Autodesk Inventor part; units mm, degrees
ref_plane "YZ Plane" through (0, 0, 0) normal (1, 0, 0) x (0, 1, 0)
ref_plane "XZ Plane" through (0, 0, 0) normal (0, 1, 0) x (-1, 0, 0)
ref_plane "XY Plane" through (0, 0, 0) normal (0, 0, 1) x (1, 0, 0)
sketch "スケッチ1" plane through (0, 0, 0) normal (1, 0, 0) x (0, 1, 0)
  line L0 (0, 0) -> (50.2, 0)
  line L1 (50.2, 0) -> (50.2, -28.2)
  line L2 (50.2, -28.2) -> (0, -28.2)
  line L3 (0, -28.2) -> (0, 0)
  line L4 (50.2, -14.1) -> (0, -14.1)
  line L5 (25.1, -28.2) -> (25.1, 0)
  circle A0 centre (25.1, -14.1) radius 15.3335
  point P0 (19.0745, 0)
  point P1 (19.0745, -28.2)
  point P2 (31.1255, -28.2)
  point P3 (31.1255, 0)
  dimension "d0" = 50.2
  dimension "d1" = 28.2
  dimension "d2" = 30.667
extrude "押し出し1" add sketch "スケッチ1" against normal blind 34
chamfer "面取り1" distance 2.5 angle 45 4 edges at (-17, 50.2, 0) (-17, 50.2, -28.2) (-17, 0, 0) (-17, 0, -28.2)
sketch "スケッチ2" plane through (-34, 0, 0) normal (-1, 0, 0) x (0, 0, 1)
  arc A0 (-28.2, 31.1255) -> (-28.2, 19.0745) centre (-14.1, 25.1) ccw
  circle A1 centre (-14.1, 25.1) radius 19.5
  point P0 (0, 0)
  dimension "d8" = 39
extrude "押し出し2" [suppressed]
sketch "スケッチ3" plane through (-36.375, 22.6, -13.1) normal (-1, 0, 0) x (0, 0, 1)
  arc A0 (-13.1, -14.4444) -> (13.1, -14.4444) centre (0, 0) ccw
  circle A1 centre (0, 0) radius 23
  point P0 (13.1, -22.6)
  dimension "d11" = 46
extrude "押し出し3" [suppressed]
sketch "スケッチ4" plane through (-42.675, 22.6, -13.1) normal (-1, 0, 0) x (0, 0, 1)
  circle A0 centre (0, 0) radius 23
  line L0 (0, 0) -> (19.85, 0)
  line L1 (19.85, 0) -> (19.85, 16.35)
  line L2 (19.85, 16.35) -> (0, 16.35)
  line L3 (0, 16.35) -> (0, 0)
  line L4 (10.6, 22.6) -> (-10.6, 22.6)
  line L5 (19.85, 0) -> (0, 0)
  line L6 (0, 0) -> (0, -14.35)
  line L7 (0, -14.35) -> (19.85, -14.35)
  line L8 (19.85, -14.35) -> (19.85, 0)
  line L9 (-19.85, 0) -> (-19.85, 16.35)
  line L10 (-19.85, 16.35) -> (0, 16.35)
  line L11 (0, -14.35) -> (-19.85, -14.35)
  line L12 (-19.85, -14.35) -> (-19.85, 0)
  point P0 (13.1, -22.6)
  point P1 (17.9744, -14.35)
  point P2 (19.85, -11.618)
  point P3 (19.85, 11.618)
  point P4 (16.1764, 16.35)
  point P5 (-16.1764, 16.35)
  point P6 (-19.85, 11.618)
  point P7 (-19.85, -11.618)
  point P8 (-17.9744, -14.35)
  dimension "d14" = 6.25
  dimension "d16" = 19.85
  dimension "d17" = 30.7
extrude "押し出し4" [suppressed]
sketch "スケッチ5" plane through (-47.675, 22.6, -13.1) normal (-1, 0, 0) x (0, 0, 1)
  line L0 (-16.1764, 16.35) -> (16.1764, 16.35)
  line L1 (0, 16.35) -> (0, -14.35)
  line L2 (17.9744, -14.35) -> (-17.9744, -14.35)
  line L3 (0, -14.35) -> (16.75, -14.35)
  line L4 (16.75, -14.35) -> (16.75, 13.35)
  line L5 (16.75, 13.35) -> (0, 13.35)
  line L6 (0, 13.35) -> (0, -14.35)
  line L7 (19.85, -11.618) -> (19.85, 11.618)
  line L8 (-16.75, -14.35) -> (-16.75, 13.35)
  line L9 (-16.75, 13.35) -> (0, 13.35)
  point P0 (13.1, -22.6)
  point P1 (19.85, -14.35)
  point P2 (19.85, 16.35)
  point P3 (-16.75, -14.35)
  dimension "d20" = 3
  dimension "d21" = 3.1
extrude "押し出し5" [suppressed]
sketch "スケッチ6" plane through (0, 0, 0) normal (1, 0, 0) x (0, 0, -1)
  line L0 (2.5, 50.2) -> (25.7, 50.2)
  line L1 (14.1, 50.2) -> (14.1, 0)
  line L2 (2.5, 0) -> (25.7, 0)
  arc A0 (0, 31.1255) -> (0, 19.0745) centre (14.1, 25.1) ccw
  line L3 (14.1, 25.1) -> (29.4335, 25.1)
  arc A1 (28.2, 19.0745) -> (28.2, 31.1255) centre (14.1, 25.1) ccw
  line L4 (14.1, 25.1) -> (24.2, 25.1)
  line L5 (24.2, 25.1) -> (24.2, 45.2)
  line L6 (24.2, 45.2) -> (14.1, 45.2)
  line L7 (14.1, 45.2) -> (14.1, 25.1)
  line L8 (24.2, 25.1) -> (24.2, 5)
  line L9 (24.2, 5) -> (14.1, 5)
  line L10 (4, 25.1) -> (4, 45.2)
  line L11 (4, 45.2) -> (14.1, 45.2)
  line L12 (4, 5) -> (14.1, 5)
  line L13 (4, 25.1) -> (4, 5)
  point P0 (0, 0)
  dimension "d24" = 20.1
  dimension "d25" = 10.1
extrude "押し出し6" cut sketch "スケッチ6" against normal blind 25
sketch "スケッチ7" plane through (-42.675, 22.6, -13.1) normal (-1, 0, 0) x (0, 0, 1)
  circle A0 centre (0, -0.4) radius 13
  line L0 (-16.75, 13.35) -> (16.75, 13.35)
  line L1 (0, 13.35) -> (0, -0.4)
  point P0 (13.1, -22.6)
  dimension "d28" = 26
  dimension "d29" = 13.75
extrude "押し出し7" [suppressed]
sketch "スケッチ8" plane through (-40.175, 22.2, -13.1) normal (-1, 0, 0) x (0, 0, 1)
  circle A0 centre (0, 0) radius 5
  point P0 (13.1, -22.2)
  dimension "d32" = 10
extrude "押し出し8" [suppressed]
sketch "スケッチ9" plane through (-40.175, 22.2, -13.1) normal (-1, 0, 0) x (0, 0, 1)
  circle A0 centre (0, 0) radius 11
  circle A1 centre (0, 0) radius 13
  point P0 (13.1, -22.2)
  point P1 (0, 11)
  point P2 (-7.7782, 7.7782)
  point P3 (-11, 0)
  point P4 (-7.7782, -7.7782)
  point P5 (0, -11)
  point P6 (7.7782, -7.7782)
  point P7 (11, 0)
  point P8 (7.7782, 7.7782)
  dimension "d35" = 22
  dimension "d38" = 360
hole "穴1" [suppressed]
sketch "スケッチ11" plane through (-37.875, 22.2, -13.1) normal (-1, 0, 0) x (0, 0, 1)
  circle A0 centre (0, 0) radius 5
  point P0 (13.1, -22.2)
hole "穴2" [suppressed]
sketch "スケッチ12" plane through (-25, 0, 0) normal (1, 0, 0) x (0, 0, -1)
  circle A0 centre (13.1, 22.2) radius 1.55
  circle A1 centre (13.1, 22.2) radius 3
  point P0 (0, 0)
  dimension "d57" = 6
extrude "押し出し10" [suppressed]
sketch "スケッチ13" plane through (-25, 0, 0) normal (1, 0, 0) x (0, 0, -1)
  circle A0 centre (5.3218, 29.9782) radius 1.25
  circle A1 centre (5.3218, 29.9782) radius 2.25
  circle A2 centre (20.8782, 29.9782) radius 1.25
  circle A3 centre (20.8782, 29.9782) radius 2.25
  circle A4 centre (5.3218, 14.4218) radius 1.25
  circle A5 centre (5.3218, 14.4218) radius 2.25
  circle A6 centre (20.8782, 14.4218) radius 1.25
  circle A7 centre (20.8782, 14.4218) radius 2.25
  point P0 (0, 0)
  dimension "d60" = 4.5
  dimension "d61" = 4.5
  dimension "d62" = 4.5
  dimension "d63" = 4.5
extrude "押し出し11" [suppressed]
sketch "スケッチ14" plane through (-25, 0, 0) normal (1, 0, 0) x (0, 0, -1)
  line L0 (4, 45.2) -> (24.2, 45.2)
  line L1 (14.1, 45.2) -> (14.1, 5)
  line L2 (24.2, 5) -> (4, 5)
  point P0 (0, 0)
  point P1 (14.1, 15.1)
  point P2 (14.1, 25.1)
  point P3 (14.1, 35.1)
  dimension "d66" = 10
  dimension "d67" = 10
hole "穴3" [suppressed]
sketch "スケッチ15" plane through (-40.175, 22.2, -13.1) normal (-1, 0, 0) x (0, 0, 1)
  point P0 (13.1, -22.2)
sketch "スケッチ16" plane through (-34, 0, 0) normal (-1, 0, 0) x (0, 0, 1)
  arc A0 (-28.2, 31.1255) -> (-28.2, 19.0745) centre (-14.1, 25.1) ccw
  circle A1 centre (-14.1, 25.1) radius 11
  point P0 (0, 0)
  point P1 (-14.1, 36.1)
  point P2 (-6.3218, 32.8782)
  point P3 (-3.1, 25.1)
  point P4 (-6.3218, 17.3218)
  point P5 (-14.1, 14.1)
  point P6 (-21.8782, 17.3218)
  point P7 (-25.1, 25.1)
  point P8 (-21.8782, 32.8782)
  dimension "d75" = 22
  dimension "d78" = 360
hole "穴4" at (-34, 32.8782, -21.8782) at (-34, 36.1, -14.1) at (-34, 32.8782, -6.3218) at (-34, 17.3218, -6.3218) at (-34, 14.1, -14.1) at (-34, 17.3218, -21.8782) direction (1, 0, 0) diameter 2.7 end through all
sketch "スケッチ17" plane through (-25, 0, 0) normal (1, 0, 0) x (0, 0, -1)
  circle A0 centre (14.1, 36.1) radius 1.35
  circle A1 centre (6.3218, 32.8782) radius 1.35
  circle A2 centre (21.8782, 32.8782) radius 1.35
  circle A3 centre (21.8782, 17.3218) radius 1.35
  circle A4 centre (14.1, 14.1) radius 1.35
  circle A5 centre (6.3218, 17.3218) radius 1.35
  point P0 (0, 0)
hole "穴5" at (-25, 36.1, -14.1) at (-25, 32.8782, -6.3218) at (-25, 32.8782, -21.8782) at (-25, 17.3218, -21.8782) at (-25, 14.1, -14.1) at (-25, 17.3218, -6.3218) direction (-1, 0, 0) diameter 4.9 depth 2.6
sketch "スケッチ18" plane through (0, 0, -25.7) normal (0, -1, 0) x (1, 0, 0)
  line L0 (-34, 0) -> (0, 0)
  line L1 (-15, 0) -> (-15, 23.2)
  line L2 (0, 23.2) -> (-34, 23.2)
  line L3 (-25, 1.5) -> (-25, 21.7)
  line L4 (-5, 0) -> (-5, 23.2)
  line L5 (-5, 11.6) -> (-15, 11.6)
  point P0 (0, 25.7)
  dimension "d94" = 10
  dimension "d95" = 10
hole "穴6" at (-15, 0, -14.1) at (-5, 0, -14.1) direction (0, 1, 0) diameter 3.3 end through all
fillet "フィレット1" radius 0.5 4 edges at (0, 45.2, -14.1) (0, 25.1, -4) (0, 25.1, -24.2) (0, 5, -14.1)
properties part number "connectpart1"
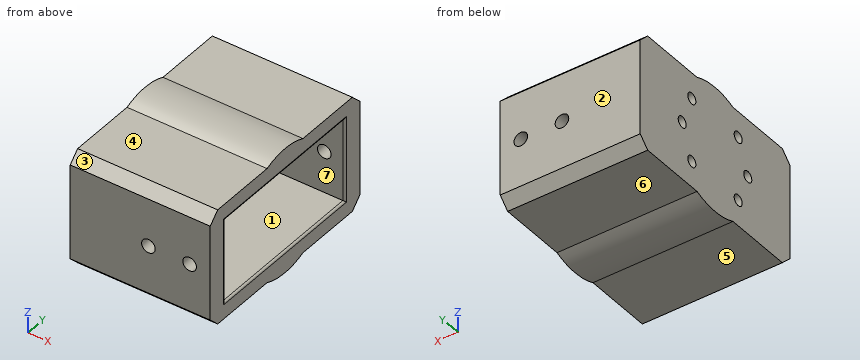
Verification items for the finished model (mm, model axes). Face numbers are marked on the shaded views. A direction names the side the tool comes from. Coordinates: 2 decimals unless noted, no trailing zeros. Order: outer loops, then holes, each group sorted by start corner. A loop starts at its lowest first (then second) coordinate and runs counter-clockwise, first axis right, second up. Notation, with made-up numbers: M 36,53 L 95,53 A25 cw 95,69 Z; hole C 55.5,84.25 d6. An arc over 180 degrees is marked long. One line per item, written item: value. Start each with the question number.
Item 1: Sectioned sample at A-A on y = 36.1. Record the cut outline in (x, z).
Item 2: Depth check by flat-ended pin: P1, Ø6, axis at x = -5, y = 18, coming from the +Z side; P2, Ø8, axis at x = -19, y = 14, coming from the +Z side; P3, Ø6, axis at y = 19, z = -9.5, coming from the +X side. Enter the tip coordinate at first touch or a pass-through.
Item 3: Access from +Z, -Z, +X, -X, +Y, -Y to the whole of each face (thin tool, end or side, straight path). Record for the marked faces 4, 5, 6 and 7.
Item 4: Sectioned sample at D-D on z = -11. Record the cut outline in (x, y).
Item 5: Sectioned sample at B-B on x = -5. Record the cut outline in (y, z).
Item 6: Mould release check, pull along Z, two halves, no side actions. Record for the marked faces 1, 2 and 3: pulls with the +Z half, pulls with the -Z half, needs draft (parallel to the pull), parting line crosses it, or undercut.
Item 7: Thickness scan on probe 1 along Y at (x, z) = (-17.5, -5); probe 2 along Z at (x, y) = (-5, 47); probe 3 along Z at (x, y) = (-12, 42.5). Record the ranges inside material, lowest first.
Item 8: Sectioned sample at C-C on x = -22. Record the cut outline in (y, z), then the cut area to 3 significant figures.
Calculated:
1. outline: M -34,-28.2 L 0,-28.2 L 0,-24.7 A0.5 ccw -0.5,-24.2 L -25,-24.2 L -25,-16.55 L -27.6,-16.55 L -27.6,-15.45 L -34,-15.45 Z; M -34,-12.75 L -27.6,-12.75 L -27.6,-11.65 L -25,-11.65 L -25,-4 L -0.5,-4 A0.5 ccw 0,-3.5 L 0,0 L -34,0 Z
2. P1: z = 0.68
2. P2: z = 0
2. P3: x = -25
3. face 4: +Z, +X, -X, -Y
3. face 5: -Z, +X, -X, -Y
3. face 6: -Z, +X, -X, +Y
3. face 7: +X
4. outline: M -34,0 L 0,0 L 0,4.5 A0.5 ccw -0.5,5 L -25,5 L -25,45.2 L -0.5,45.2 A0.5 ccw 0,45.7 L 0,50.2 L -34,50.2 Z
5. outline: M 0,-25.7 L 2.5,-28.2 L 19.07,-28.2 A15.33 ccw 31.13,-28.2 L 47.7,-28.2 L 50.2,-25.7 L 50.2,-15.75 L 45.2,-15.75 L 45.2,-24.2 L 5,-24.2 L 5,-15.75 L 0,-15.75 Z; M 0,-12.45 L 5,-12.45 L 5,-4 L 45.2,-4 L 45.2,-12.45 L 50.2,-12.45 L 50.2,-2.5 L 47.7,0 L 31.13,0 A15.33 ccw 19.07,0 L 2.5,0 L 0,-2.5 Z
6. face 1: undercut
6. face 2: needs draft
6. face 3: pulls with the +Z half
7. probe 1: 0 to 5, 45.2 to 50.2
7. probe 2: -28.2 to -15.75, -12.45 to 0
7. probe 3: -28.2 to -24.2, -4 to 0
8. outline: M 0,-25.7 L 2.5,-28.2 L 19.07,-28.2 A15.33 ccw 31.13,-28.2 L 47.7,-28.2 L 50.2,-25.7 L 50.2,-2.5 L 47.7,0 L 31.13,0 A15.33 ccw 19.07,0 L 2.5,0 L 0,-2.5 Z; hole M 5,-24.2 L 45.2,-24.2 L 45.2,-4 L 5,-4 Z
8. area: 611 mm^2
